The model under review builds one solid part; all positions refer to its coordinate system, in mm. Face numbers are marked on the shaded views. A direction names the side the tool comes from. Round coordinates to 2 decimals unless told otherwise and drop trailing zeros. Loops run counter-clockwise (first coordinate to the right, second up) from the corner with the lowest first, then second, coordinate; pieces in that order, holes last. Notation, with made-up numbers: (-13, 20) -> (40, 20) arc R11 cw to (40, 25) -> close; hole circle Ø1 at (-9, 40.25). An arc over 180 degrees is marked (long way). Write each question's results on one line, items separated by ' | '. Start each with the question number.
Item 1: Tool access review of the marked faces 1 and 2: name each direction out of +Z, -Z, +X, -X, +Y, -Y from which nothing blocks a thin tool from reaching the whole face with its end or side.
Item 2: For L1, parallel to X at y = -16, z = 0; L2, parallel to Z at x = 3.25, y = 0.25, list the stretches that pass through material, from the lowest coordinate up. Write a range as from..to.
Item 3: Clearance check with flat-ended pins moving along their axes: pin 1 Ø3 at (y, z) = (-4.5, 6.5) entering from +X; pin 2 Ø1 at (x, y) = (-1.5, -11.5) entering from -Z; pin 3 Ø2 at (x, y) = (-6, -11) entering from -Z. State where each tip first meets the part, or that it passes through.
Item 4: We need section A-A (y = -9.5). Give the boundary of the cut face in (x, z).
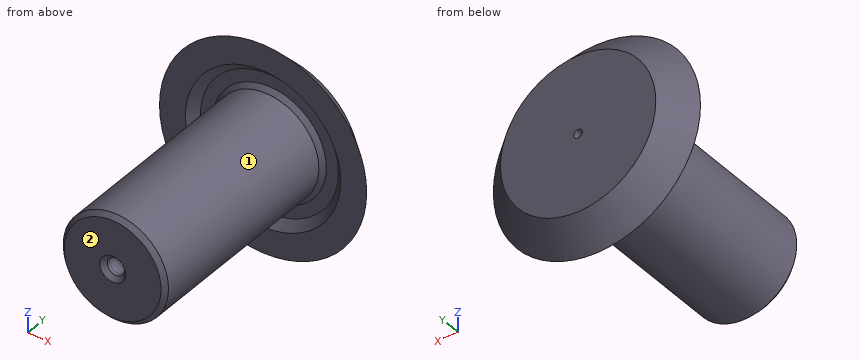
from build123d import *

# Parameters (mm, degrees)
CHAMFER2_SIZE = 0.5


with BuildPart() as part:
    # Sketch2 → Revolve1 (revolve)
    with BuildSketch(Plane.XY):
        with BuildLine():
            Line((12, 0), (9, 3))
            Line((9, 3), (1, 3))
            Line((1, 3), (0.5, 3))
            Line((0.5, 3), (0.5, 2.310660172))
            ThreePointArc((0.5, 2.310660172), (0.557090351, 2.023647598), (0.719669914, 1.780330086))
            Line((0.719669914, 1.780330086), (0.780330086, 1.719669914))
            ThreePointArc((0.780330086, 1.719669914), (0.942909649, 1.476352402), (1, 1.189339828))
            Line((1, 1.189339828), (1, -20.881966011))
            ThreePointArc((1, -20.881966011), (0.912870929, -21.290214302), (0.666666667, -21.627322004))
            ThreePointArc((0.666666667, -21.627322004), (0.5, -22), (0.666666667, -22.372677996))
            ThreePointArc((0.666666667, -22.372677996), (0.912870929, -22.709785698), (1, -23.118033989))
            Line((1, -23.118033989), (1, -24))
            Line((1, -24), (6.1, -24))
            Line((6.1, -24), (6.1, 1))
            Line((6.1, 1), (8, 1))
            Line((8, 1), (9, 0))
            Line((9, 0), (12, 0))
        make_face()
    revolve(axis=Axis((0, -747.512282571, 0), (0, 1, 0)))

    # Chamfer2
    chamfer2_edges = [part.edges().sort_by_distance(p)[0] for p in [
        (-1, -24, 0),
        (-6.1, -24, 0),
        (-6.1, 1, 0),
    ]]
    chamfer(chamfer2_edges, length=CHAMFER2_SIZE)


solid = part.part
Here are the results:
1) face 1: -Y | face 2: +Z, -Z, +X, -X, -Y
2) L1: x = -6.1..-1, 1..6.1 | L2: z = -11.29..-8.12, -5.16..5.16, 8.12..11.29
3) pin 1: stops at x = 3.49 | pin 2: stops at z = -6.02 | pin 3: stops at z = -3.49
4) outline: circle Ø12.2 at (0, 0); hole circle Ø2 at (0, 0)
